```python
from build123d import *

# Parameters (mm, degrees)
SKETCH1_R           = 48
BOSS_EXTRUDE1_DEPTH = 20
FILLET1_R           = 4
SKETCH2_R           = 7.089026355
CUT_EXTRUDE1_DEPTH  = 4
FILLET3_R           = 1
CHAMFER1_SIZE       = 0.5


with BuildPart() as part:
    # Sketch1 → Boss-Extrude1 (new body)
    with BuildSketch(Plane.XY):
        Circle(SKETCH1_R)
    extrude(amount=-BOSS_EXTRUDE1_DEPTH)

    # Fillet1
    fillet1_edges = [part.edges().sort_by_distance(p)[0] for p in [
        (-48, 0, 0),
    ]]
    fillet(fillet1_edges, radius=FILLET1_R)

    # Sketch2 → Cut-Extrude1 (cut)
    with BuildSketch(Plane.XY):
        with Locations((0, 33.015746337)):
            Circle(SKETCH2_R)
    extrude(amount=-CUT_EXTRUDE1_DEPTH, mode=Mode.SUBTRACT)

    # Fillet3
    fillet3_edges = [part.edges().sort_by_distance(p)[0] for p in [
        (-7.089026355, 33.015746337, 0),
    ]]
    fillet(fillet3_edges, radius=FILLET3_R)

    # Chamfer1
    chamfer1_edges = [part.edges().sort_by_distance(p)[0] for p in [
        (-7.089026355, 33.015746337, -4),
    ]]
    chamfer(chamfer1_edges, length=CHAMFER1_SIZE)


solid = part.part
```
Verification items for the finished model (mm, model axes). A direction names the side the tool comes from. Coordinates: 2 decimals unless noted, no trailing zeros. Order: outer loops, then holes, each group sorted by start corner. A loop starts at its lowest first (then second) coordinate and runs counter-clockwise, first axis right, second up. Notation, with made-up numbers: (30, -34) -> (62, -34) arc R15 cw to (62, -30) -> close; hole circle Ø2 at (27, 3.25). An arc over 180 degrees is marked (long way). Answer as CSV lines item,"result". Start each with the question number.
1) Cross-section at B-B, the plane z = -12. Record the boundary of the cut face in (x, y), then the cut area to 3 significant figures.
2) Material ranges on L1, parallel to X at y = 1, z = -6; L2, parallel to Y at x = 0, z = -1.85; L3, parallel to Y at x = 0, z = -2.4, recorded low to high. Write a range as [from, to].
3) Cross-section at A-A, the plane x = 0. Record the boundary of the cut face in (y, z), then the cut area to 3 significant figures.
4) Release check for a two-part mould opening along Y. For faces 3 (the face through (-1, 1, 0)), 4 (the face through (-47.954, 2.11, -11.888)), 5 (the face through (-0.923, 40.044, -2.232)) record: released by +Y, released by -Y, zero draft, split by the parting line, or undercut.
5) Set-up check for faces 1 (the face through (0, 33, -4)), 2 (the face through (-1, 1, -20)): record each of +Z, -Z, +X, -X, +Y, -Y from which the full face is reachable in a straight line by a thin tool's end or side.
6) Gauge pin test, flat ends, axial feed: pin 1 Ø12 at (y, z) = (34.5, -6.5) entering from +X; pin 2 Ø1 at (y, z) = (6.5, -6.5) entering from -X; pin 3 Ø5 at (x, z) = (13, -14) entering from +Y; pin 4 Ø22.5 at (x, y) = (0, 33.02) entering from +Z. Record the tip position at first contact, or that the pin passes through.
Conclusion:
1,outline,"circle Ø96 at (0, 0)"
1,area,"7,240 mm²"
2,L1,"x = [-47.99, 47.99]"
2,L2,"y = [-47.37, 25.93], [40.1, 47.37]"
2,L3,"y = [-47.67, 25.93], [40.1, 47.67]"
3,outline,"(-48, -20) -> (48, -20) -> (48, -4) arc R4 ccw to (44, 0) -> (41.1, 0) arc R1 ccw to (40.1, -1) -> (40.1, -3.5) -> (39.6, -4) -> (26.43, -4) -> (25.93, -3.5) -> (25.93, -1) arc R1 ccw to (24.93, 0) -> (-44, 0) arc R4 ccw to (-48, -4) -> close"
3,area,"1,860 mm²"
4,face 3,"zero draft"
4,face 4,"split by the parting line"
4,face 5,"undercut"
5,face 1,"+Z"
5,face 2,"-Z, +X, -X, +Y, -Y"
6,pin 1,"stops at x = 38.62"
6,pin 2,"stops at x = -47.62"
6,pin 3,"stops at y = 46.84"
6,pin 4,"stops at z = 0"
